from build123d import *

# Parameters (mm, degrees)
F0_W     = 290
F0_H     = 314
F1_DEPTH = 18
F3_DEPTH = 5
F4_R     = 17.99999


# Not quite as in the source:
# - a fillet or chamfer is up to 0.001 mm smaller than in the source, because OpenCascade refuses the exact size


with BuildPart() as f1:
    # F0 (on Right) → F1 (new body)
    with BuildSketch(Plane.YZ):
        Rectangle(F0_W, F0_H)
    extrude(amount=F1_DEPTH)

    # F2 (on face) → F3 (cut)
    with BuildSketch(Plane(origin=(0, 0, 0), x_dir=(0, -1, 0), z_dir=(-1, 0, 0))):
        with BuildLine():
            Line((28.5, 9), (-28.5, 9))
            ThreePointArc((-28.5, 9), (-37.5, 0), (-28.5, -9))
            Line((-28.5, -9), (28.5, -9))
            ThreePointArc((28.5, -9), (37.5, 0), (28.5, 9))
        make_face()
    extrude(amount=-F3_DEPTH, mode=Mode.SUBTRACT)

    # F4 (radius 18 in the source; OpenCascade refuses exactly that, so slightly less here)
    f4_edges = [f1.edges().sort_by_distance(p)[0] for p in [
        (0, 145, 0),
    ]]
    fillet(f4_edges, radius=F4_R)


solid = f1.part
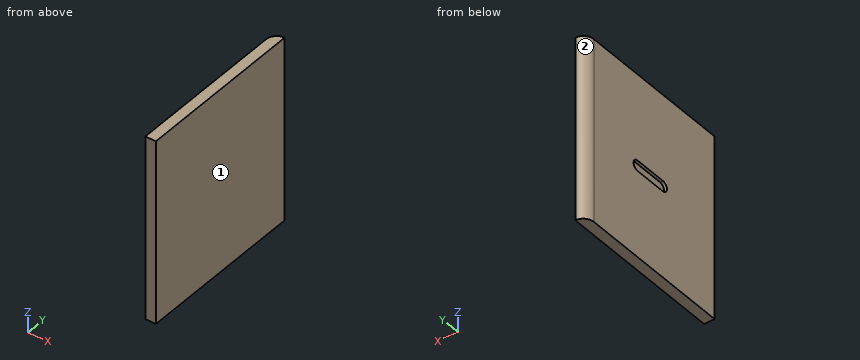
The model under review builds one solid part; all positions refer to its coordinate system, in mm. Face numbers are marked on the shaded views. Give positions to 0.01 mm unless a question says otherwise; leave off trailing zeros. Order: outer loops, then holes, each group sorted by start corner. A loop starts at its lowest first (then second) coordinate and runs counter-clockwise, first axis right, second up. Notation, with made-up numbers: M 10.5,-28 L 44.5,-28 A18 ccw 44.5,1 Z; hole C 28,64 d8. An arc over 180 degrees is marked long. Use one line per item in the form item = value. Start each with the question number.
Item 1: The part is to be moulded in two halves that separate along X. For the marked faces 1 and 2, say which applies: pulls with the +X half, pulls with the -X half, needs draft (parallel to the pull), parting line crosses it, or undercut.
Item 2: We need section B-B on y = 13. Give the boundary of the cut face in (x, z).
Item 3: To check wall thickness, follow line 1 along Z through (x, y) = (4, -26.5); line 2 along Y through (x, z) = (3, -68.5); line 3 along Y through (x, z) = (16.25, 76.5). State the ranges of each line that lie inside material, in increasing order. Write a range as from..to.
Item 4: Insertion check: pin 1 Ø10 at (x, z) = (2.5, -48.5) entering from +Y; pin 2 Ø3 at (x, z) = (2, -24) entering from +Y. Each pin has a flat end and moves straight along its axis. Give the tip position at first contact, or say it passes through.
Completed:
q1.face_1 = pulls with the +X half
q1.face_2 = pulls with the -X half
q2.outline = M 0,-157 L 18,-157 L 18,157 L 0,157 L 0,9 L 5,9 L 5,-9 L 0,-9 Z
q3.line_1 = -157..-9, 9..157
q3.line_2 = -145..136.95
q3.line_3 = -145..144.91
q4.pin_1 = 141.62
q4.pin_2 = 137.67
